CAD build for the part. Positions are in the model's coordinates, mm. A direction names the side the tool comes from. Give positions to 0.01 mm unless a question says otherwise; leave off trailing zeros. Loops run counter-clockwise (first coordinate to the right, second up) from the corner with the lowest first, then second, coordinate; pieces in that order, holes last.
```python
from build123d import *

# Parameters (mm, degrees)
F0_W     = 127
F0_H     = 50.8
F1_DEPTH = 12.7
F2_R     = 7.9375
F2_R_2   = 6.35
F2_W     = 12.7
F2_H     = 25.4
F3_DEPTH = 38.1
F4_W     = 12.7
F4_H     = 8.466582
F4_H_2   = 8.46582
F5_DEPTH = 12.7
F6_R     = 6.34999
F7_R     = 3.175
F8_DEPTH = 25.4


# Not quite as in the source:
# - a fillet or chamfer is up to 0.001 mm smaller than in the source, because OpenCascade refuses the exact size


with BuildPart() as f1:
    # F0 (on Top) → F1 (new body)
    with BuildSketch(Plane.XY):
        with Locations((-63.5, 25.4)):
            Rectangle(F0_W, F0_H)
    extrude(amount=F1_DEPTH)

    # F2 (on face) → F3 (join)
    with BuildSketch(Plane.XY.offset(12.7)):
        with Locations((-25.4, 25.4)):
            Circle(F2_R)
        with Locations((-25.4, 25.4)):
            Circle(F2_R_2, mode=Mode.SUBTRACT)
        with Locations((-82.55, 25.4)):
            Rectangle(F2_W, F2_H)
    extrude(amount=F3_DEPTH)

    # F4 (on face) → F5 (join)
    with BuildSketch(Plane.XY.offset(50.8)):
        with Locations((-82.55, 33.866709)):
            Rectangle(F4_W, F4_H)
        with Locations((-82.55, 16.93291)):
            Rectangle(F4_W, F4_H_2)
    extrude(amount=F5_DEPTH)

    # F6 (radius 6.35 in the source; OpenCascade refuses exactly that, so slightly less here)
    f6_edges = [f1.edges().sort_by_distance(p)[0] for p in [
        (-88.9, 33.866709, 63.5),
        (-88.9, 16.93291, 63.5),
        (-76.2, 33.866709, 63.5),
        (-76.2, 16.93291, 63.5),
        (-88.9, 25.399619, 50.8),
        (-76.2, 25.399619, 50.8),
    ]]
    fillet(f6_edges, radius=F6_R)

    # F7 (on face) → F8 (cut)
    with BuildSketch(Plane(origin=(0, 38.1, 0), x_dir=(-1, 0, 0), z_dir=(0, 1, 0))):
        with Locations((82.55, 57.15)):
            Circle(F7_R)
    extrude(amount=-F8_DEPTH, mode=Mode.SUBTRACT)


solid = f1.part
```
1. Saw through at A-A, the plane z = 18. Count the separate pieces of the cut face and the enclosed holes in it, and give its area (3 significant figures).
Responses:
separate pieces: 2
enclosed holes: 1
area: 394 mm2
2. Probe line 1 along X through (y, z) = (25.5, 15.5); line 2 along X through (y, z) = (28.5, 28); line 3 along Z through (x, y) = (-115, 5). List the from-to ranges inside material, lowest first.
Responses:
line 1: x = -88.9 to -76.2, -33.34 to -31.75, -19.05 to -17.46
line 2: x = -88.9 to -76.2, -32.71 to -30.94, -19.86 to -18.09
line 3: z = 0 to 12.7
3. Tool access for faces 5 (the face through (-83, 38.1, 38)), 6 (the face through (-76.2, 25, 35)), 7 (the face through (-88.9, 25, 35)): list every direction of +Z, -Z, +X, -X, +Y, -Y with a clear straight run to the whole face (end or side of a thin tool).
Responses:
face 5: +Z, +X, -X, +Y
face 6: +Z, +Y, -Y
face 7: +Z, -X, +Y, -Y
4. Saw through at B-B, the plane x = -25.4. List the corners of the cut face in (y, z), and give its area (3 significant figures).
Responses:
outline: (0, 0) - (50.8, 0) - (50.8, 12.7) - (33.34, 12.7) - (33.34, 50.8) - (31.75, 50.8) - (31.75, 12.7) - (19.05, 12.7) - (19.05, 50.8) - (17.46, 50.8) - (17.46, 12.7) - (0, 12.7) - close
area: 766 mm2
5. Saw through at D-D, the plane x = -11. List the corners of the cut face in (y, z).
Responses:
outline: (0, 0) - (50.8, 0) - (50.8, 12.7) - (0, 12.7) - close
6. Drop flat-ended pins along their axis: pin 1 (10 mm diameter, centred on x = -80, z = 49, fed in from -Y); pin 2 (20.5 mm diameter, centred on y = 31, z = 29.5, fed in from -X); pin 3 (8 mm diameter, centred on x = -24.5, y = 24.5, fed in from +Z); pin 4 (8 mm diameter, centred on x = -89, y = 38, fed in from -Z). Give the stop position or say it passes through.
Responses:
pin 1: stops at y = 12.7
pin 2: stops at x = -88.9
pin 3: stops at z = 12.7
pin 4: stops at z = 0
7. Pull direction Y, two halves, no side cores. Call faces 1 (the face through (-87.09, 16.99, 61.59)), 2 (the face through (-78.11, 25.46, 48.99)), 3 (the face through (-82.6, 29.633, 53.8)), 4 (the face through (-83, 12.7, 38)): released by +Y, released by -Y, zero draft, split by the parting line, or undercut.
Responses:
face 1: zero draft
face 2: undercut
face 3: undercut
face 4: released by -Y
